Here's the drawing with two shaded views (mm, measured from the low corner). I have some questions. A direction names the side the tool comes from. Give positions to 0.01 mm unless a question says otherwise; leave off trailing zeros. Order: outer loops, then holes, each group sorted by start corner. A loop starts at its lowest first (then second) coordinate and runs counter-clockwise, first axis right, second up. Notation, with made-up numbers: M 19.25,-19.75 L 30.25,-19.75 A20 ccw 30.25,5.25 Z; hole C -36,8 d4. An arc over 180 degrees is marked long. Use a Markdown table: item, result. Add a question column.
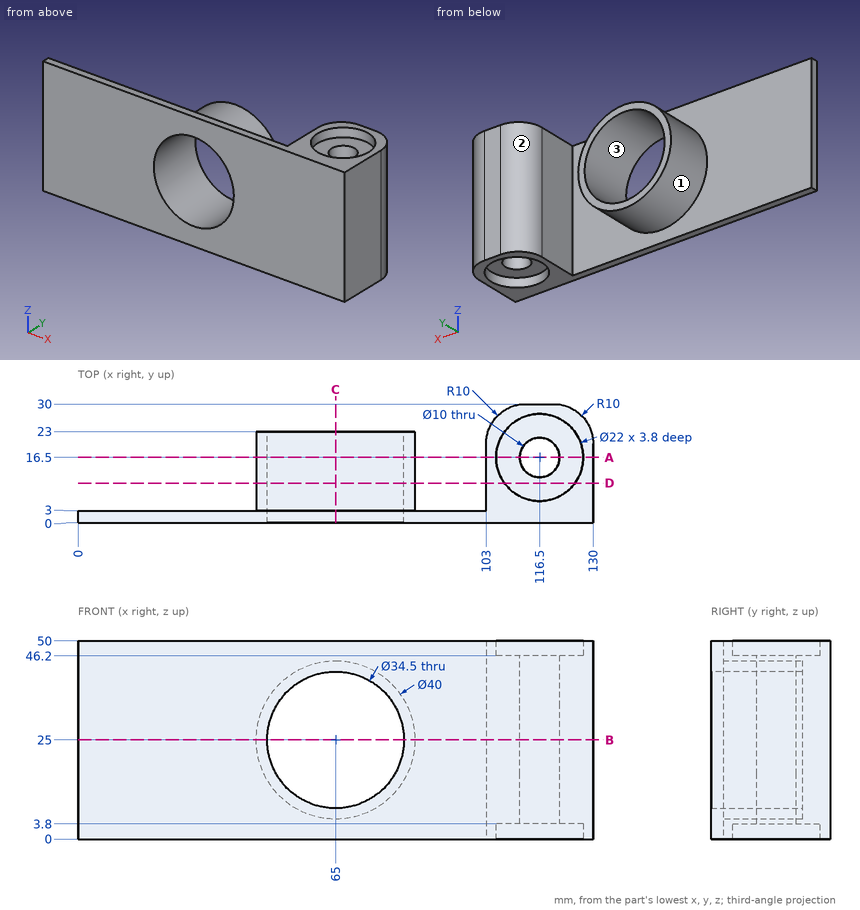
1. On a 3-axis mill with a long thin cutter (end or side, diameter ignored), from which of +Z, -Z, +X, -X, +Y, -Y can I reach the whole of each face in a straight line? I mean the marked faces 1, 2 and 3. Say none if no direction works.
2. If we section it at C-C, the plane x = 65: List the corners of the cut face in (y, z) for me.
3. If we section it at A-A, the plane y = 16.5: List the corners of the cut face in (x, z) for me.
4. I need wall thicknesses on L1, parallel to X at y = 16.5, z = 1.45; L2, parallel to X at y = 6.75, z = 25; L3, parallel to X at y = 4.25, z = 17.5. Which ranges of each line are inside material? Lowest first, please. Write a range as [from, to].
5. Will these pins go through, and if not, where does the flat tip stop? pin 1 (5 mm diameter, centred on y = 10, z = 37, fed in from -X); pin 2 (1.5 mm diameter, centred on x = 50.5, z = 14.5, fed in from +Y); pin 3 (6.5 mm diameter, centred on x = 119.5, y = 17.5, fed in from +Z); pin 4 (9 mm diameter, centred on x = 116.5, y = 16.5, fed in from -Z).
6. If we section it at D-D, the plane y = 10: List the corners of the cut face in (x, z) for me, then the cut area to 3 significant figures.
7. If we section it at B-B, the plane z = 25: List the corners of the cut face in (x, y) for me, then the cut area to 3 significant figures.
Geometry results:
| question | item | result |
|---|---|---|
| 1 | face 1 | +Y |
| 1 | face 2 | +Z, -Z, +Y |
| 1 | face 3 | +Y, -Y |
| 2 | outline | M 0,0 L 3,0 L 3,5 L 23,5 L 23,7.75 L 0,7.75 Z; M 0,42.25 L 23,42.25 L 23,45 L 3,45 L 3,50 L 0,50 Z |
| 3 | outline | C 65,25 d40; M 103,0 L 105.5,0 L 105.5,3.8 L 111.5,3.8 L 111.5,46.2 L 105.5,46.2 L 105.5,50 L 103,50 Z; M 121.5,3.8 L 127.5,3.8 L 127.5,0 L 130,0 L 130,50 L 127.5,50 L 127.5,46.2 L 121.5,46.2 Z; hole C 65,25 d34.5 |
| 4 | L1 | x = [103, 105.5], [127.5, 130] |
| 4 | L2 | x = [45, 47.75], [82.25, 85], [103, 130] |
| 4 | L3 | x = [46.46, 49.47], [80.53, 83.54], [103, 130] |
| 5 | pin 1 | stops at x = 47.4 |
| 5 | pin 2 | stops at y = 23 |
| 5 | pin 3 | stops at z = 46.2 |
| 5 | pin 4 | passes through |
| 6 | outline | C 65,25 d40; M 103,0 L 107.63,0 L 107.63,3.8 L 125.37,3.8 L 125.37,0 L 130,0 L 130,50 L 125.37,50 L 125.37,46.2 L 107.63,46.2 L 107.63,50 L 103,50 Z; hole C 65,25 d34.5 |
| 6 | area | 1,540 mm^2 |
| 7 | outline | M 0,0 L 47.75,0 L 47.75,23 L 45,23 L 45,3 L 0,3 Z; M 82.25,0 L 130,0 L 130,20 A10 ccw 120,30 L 113,30 A10 ccw 103,20 L 103,3 L 85,3 L 85,23 L 82.25,23 Z; hole C 116.5,16.5 d10 |
| 7 | area | 1,000 mm^2 |
